Build history of the part. All positions in model axes, mm. A direction names the side the tool comes from. Give positions to 0.01 mm unless a question says otherwise; leave off trailing zeros. Write each loop counter-clockwise with the first axis right and the second up, starting at its lowest first coordinate (ties: lowest second). Pieces come first, ordered by that corner, then holes. Notation, with made-up numbers: (-33.5, 30) -> (15.5, 30) arc R27 ccw to (15.5, 63) -> close; hole circle Ø10 at (84.5, -24.5). An arc over 180 degrees is marked (long way). One line per question, with ' | ' between items. Start each with the question number.
(1) Band-saw the part on C-C, the plane z = 27. Give the cut face in (x, y), and give its area (3 significant figures).
(2) Band-saw the part on A-A, the plane x = 9.25. Give the cut face in (y, z).
(3) Pin check, flat tips, straight feed: P1, Ø1.5, axis at x = 7, z = 13, coming from the +Y side; P2, Ø10, axis at y = 5, z = 16, coming from the +X side; P3, Ø7, axis at x = -0.5, y = -1.5, coming from the -Z side. Stop position of each tip, or through.
(4) Tool access for faces 4 (the cylindrical face through (-8.59, 0.38, 14.35)), 5 (the flat face through (8.6, -4, 2)), 6 (the flat face through (8.6, 4, 2)), 7 (the cylindrical face through (3.35, -6.43, 11.63)): list every direction of +Z, -Z, +X, -X, +Y, -Y with a clear straight run to the whole face (end or side of a thin tool).
(5) Band-saw the part on B-B, the plane z = 12.5. Give the cut face in (x, y), and give its area (3 significant figures).
(6) Pull direction X, two halves, no side cores. Call faces 1 (the flat face through (2, -2, 29.1)), 2 (the flat face through (0, 0, 26.6)), 3 (the flat face through (11.6, 0, 4)): released by +X, released by -X, zero draft, split by the parting line, or undercut.
(7) Drill centre lines: probe 1 along Y at (x, z) = (0, 8); probe 2 along Y at (x, z) = (0.25, 28.5). Where is each one in solid material? Low to high. Write a range as from..to.
from build123d import *

# Parameters (mm, degrees)
F0_R         = 8.6
F0_R_2       = 7.25
F1_DEPTH     = 29.1
F2_R         = 8.6
F3_DEPTH     = 2.5
F4_R         = 3
F5_R         = 2.3
F6_DEPTH     = 2
F7_DEPTH     = 2
F8_R         = 3.5
F9_DEPTH     = 2.2
F10_R        = 2
F12_DEPTH    = 4.5
F13_T1_DEPTH = 22.4300979278
F14_R        = 1


# Not quite as in the source:
# - a fillet or chamfer that OpenCascade refuses, or shapes differently, is made with other operations: its cross-section is extruded or revolved along the edge and cut away or added


with BuildPart() as f1:
    # F0 (on Top) → F1 (new body)
    with BuildSketch(Plane.XY):
        Circle(F0_R)
        Circle(F0_R_2, mode=Mode.SUBTRACT)
    extrude(amount=F1_DEPTH)

    # F2 (on face) → F3 (join)
    with BuildSketch(Plane.XY.offset(29.1)):
        Circle(F2_R)
    extrude(amount=-F3_DEPTH)

    # F4
    f4_edges = [f1.edges().sort_by_distance(p)[0] for p in [
        (-7.25, 0, 26.6),
    ]]
    fillet(f4_edges, radius=F4_R)

    # F5 (on face) → F6 (join)
    with BuildSketch(Plane.XY.offset(29.1)):
        Circle(F5_R)
    extrude(amount=F6_DEPTH)

    # F5 (on face) → F7 (join)
    with BuildSketch(Plane.XY.offset(29.1)):
        Circle(F5_R)
    extrude(amount=-F7_DEPTH)

    # F8 (on face) → F9 (join)
    with BuildSketch(Plane.XY.offset(31.1)):
        Circle(F8_R)
    extrude(amount=F9_DEPTH)

    # F10
    f10_edges = [f1.edges().sort_by_distance(p)[0] for p in [
        (-3.5, 0, 33.3),
    ]]
    fillet(f10_edges, radius=F10_R)

    # F11 (on face) → F12 (join)
    with BuildSketch(Plane(origin=(0, 0, 0), x_dir=(1, 0, 0), z_dir=(0, 0, -1))):
        Polygon((8.6, -3.5), (8.6, 0), (7.3356842622, 0), (7.3356842622, -6), (8.6, -6), align=None)
        Polygon((7.3356842622, 0), (8.6, 0), (8.6, 0.5253988202), (8.6, 3.5), (8.6, 6), (7.3356842622, 6), align=None)
        Polygon((8.7317479774, 0), (8.6, 0), (8.6, -3.5), (11.6, -3.5), (11.6, 0), align=None)
        with BuildLine():
            Line((7.3356842622, -6), (7.3356842622, 0))
            Line((7.3356842622, 0), (7.3356842622, 6))
            Line((7.3356842622, 6), (6.1521958246, 6))
            Line((6.1521958246, 6), (6.1521958246, 3.8678361166))
            ThreePointArc((6.1521958246, 3.8678361166), (7.267026193, 0), (6.1521958246, -3.8678361166))
            Line((6.1521958246, -3.8678361166), (6.1521958246, -6.0092001577))
            Line((6.1521958246, -6.0092001577), (7.3356842622, -6.0092001577))
            Line((7.3356842622, -6.0092001577), (7.3356842622, -6))
        make_face()
        Polygon((8.6, 3.5), (8.6, 0.5253988202), (8.7317479774, 0.5253988202), (8.7317479774, 0), (11.6, 0), (11.6, 3.5), align=None)
    extrude(amount=-F12_DEPTH)

    # F13: chamfer of 3 on 1 edges, made by hand

    # F13_s2 → F13_t1 (cut)
    with BuildSketch(Plane.XZ.offset(-11.2150489639)):
        Polygon((8.6, 0), (11.6, 3), (11.6, 0), align=None)
    extrude(amount=F13_T1_DEPTH, mode=Mode.SUBTRACT)

    # F14
    f14_edges = [f1.edges().sort_by_distance(p)[0] for p in [
        (8.6, 6, 2.25),
        (8.6, -6, 2.25),
    ]]
    fillet(f14_edges, radius=F14_R)


solid = f1.part
Results:
1) outline: circle Ø17.2 at (0, 0) | area: 232 mm²
2) outline: (-3.5, 0.65) -> (3.5, 0.65) -> (3.5, 4.5) -> (-3.5, 4.5) -> close
3) P1: stops at y = 5.91 | P2: stops at x = 8.6 | P3: stops at z = 26.48
4) face 4: +Z | face 5: +Z, -Z, +X, -Y | face 6: +Z, -Z, +X, +Y | face 7: -Z
5) outline: circle Ø17.2 at (0, 0); hole circle Ø14.5 at (0, 0) | area: 67.2 mm²
6) face 1: zero draft | face 2: undercut | face 3: released by +X
7) probe 1: y = -8.6..-7.25, 7.25..8.6 | probe 2: y = -8.6..8.6
